Autodesk Inventor part; units mm, degrees
ref_plane "YZ Plane" through (0, 0, 0) normal (1, 0, 0) x (0, 1, 0)
ref_plane "XZ Plane" through (0, 0, 0) normal (0, 1, 0) x (-1, 0, 0)
ref_plane "XY Plane" through (0, 0, 0) normal (0, 0, 1) x (1, 0, 0)
sketch "Sketch1" plane through (0, 0, 0) normal (0, 0, 1) x (1, 0, 0)
  line L0 (-28.9445, 15.5893) -> (396.7701, 15.5893) construction
  line L1 (396.7701, 15.5893) -> (396.7701, -233.6482) construction
  line L2 (396.7701, -233.6482) -> (-28.9445, -233.6482) construction
  line L3 (-28.9445, -233.6482) -> (-28.9445, 15.5893) construction
  line L4 (-26.909, 14.1495) -> (398.8056, 14.1495) construction
  line L5 (398.8056, 14.1495) -> (398.8056, -235.0879) construction
  line L6 (398.8056, -235.0879) -> (-26.909, -235.0879) construction
  line L7 (-26.909, -235.0879) -> (-26.909, 14.1495) construction
  point P0 (0, 0)
sketch "Sketch2" plane through (0, 0, 0) normal (0, 0, 1) x (1, 0, 0)
  circle A0 centre (97.339, -21.1948) radius 15.8949
  circle A1 centre (275.5323, -21.1948) radius 15.8949
  circle A2 centre (275.5323, -200.173) radius 15.8949
  circle A3 centre (97.339, -200.173) radius 15.8949
  circle A4 centre (185.2582, -110.6839) radius 89.4891
  line L0 (65.9394, 9.4199) -> (306.932, 9.4199)
  line L1 (306.932, 9.4199) -> (306.932, -229.2178)
  line L2 (306.932, -229.2178) -> (65.9394, -229.2178)
  line L3 (65.9394, -229.2178) -> (65.9394, 9.4199)
  point P0 (0, 0)
extrude "Extrusion1" add sketch "Sketch2" along normal blind 6.35
properties part number "Ball grabber bearing mount2"
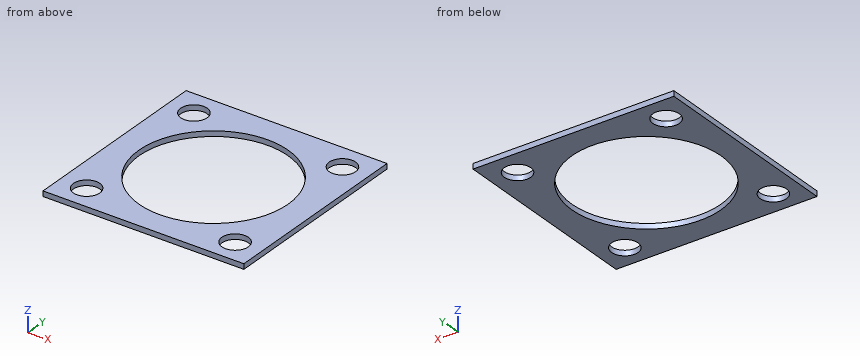
Here's how the part is built. I have some questions about the finished solid (model axes, mm). Coordinates: 2 decimals unless noted, no trailing zeros. Write each loop counter-clockwise with the first axis right and the second up, starting at its lowest first coordinate (ties: lowest second). Pieces come first, ordered by that corner, then holes. Notation, with made-up numbers: (-7, 41.5) -> (23, 41.5) arc R20 ccw to (23, 53.5) -> close; hole circle Ø10 at (10.5, 15.25). An arc over 180 degrees is marked (long way). Use a Markdown table: item, result. Add a question column.
(1) If we section it at A-A, the plane y = -47: Write out the boundary of the cut face in (x, z), and give its area (3 significant figures).
(2) Please list where these lines run through material, in increasing order: line 1 (X direction, y = -13.5, z = 2.25); line 2 (Y direction, x = 105.5, z = 1.25); line 3 (X direction, y = -202, z = 5).
(3) If we section it at B-B, the plane x = 126: Write out the boundary of the cut face in (y, z).
(4) If we section it at D-D, the plane z = 4.25: Write out the boundary of the cut face in (x, y).
(5) If we section it at C-C, the plane y = -213: Write out the boundary of the cut face in (x, z), and give its area (3 significant figures).
Outcome:
| question | item | result |
|---|---|---|
| 1 | outline | (65.94, 0) -> (122.39, 0) -> (122.39, 6.35) -> (65.94, 6.35) -> close; (248.13, 0) -> (306.93, 0) -> (306.93, 6.35) -> (248.13, 6.35) -> close |
| 1 | area | 732 mm^2 |
| 2 | line 1 | x = 65.94 to 83.43, 111.25 to 261.62, 289.44 to 306.93 |
| 2 | line 2 | y = -229.22 to -213.81, -186.53 to -151.27, -70.1 to -34.83, -7.55 to 9.42 |
| 2 | line 3 | x = 65.94 to 81.55, 113.13 to 259.74, 291.32 to 306.93 |
| 3 | outline | (-229.22, 0) -> (-177.74, 0) -> (-177.74, 6.35) -> (-229.22, 6.35) -> close; (-43.63, 0) -> (9.42, 0) -> (9.42, 6.35) -> (-43.63, 6.35) -> close |
| 4 | outline | (65.94, -229.22) -> (306.93, -229.22) -> (306.93, 9.42) -> (65.94, 9.42) -> close; hole circle Ø31.79 at (97.34, -200.17); hole circle Ø31.79 at (97.34, -21.19); hole circle Ø178.98 at (185.26, -110.68); hole circle Ø31.79 at (275.53, -200.17); hole circle Ø31.79 at (275.53, -21.19) |
| 5 | outline | (65.94, 0) -> (87.95, 0) -> (87.95, 6.35) -> (65.94, 6.35) -> close; (106.73, 0) -> (266.15, 0) -> (266.15, 6.35) -> (106.73, 6.35) -> close; (284.92, 0) -> (306.93, 0) -> (306.93, 6.35) -> (284.92, 6.35) -> close |
| 5 | area | 1,290 mm^2 |
